Check sheet for the modelled part. Datum: model origin and axes. Units: mm. Give positions to 0.01 mm unless a question says otherwise; leave off trailing zeros. Loops run counter-clockwise (first coordinate to the right, second up) from the corner with the lowest first, then second, coordinate; pieces in that order, holes last. Notation, with made-up numbers: (-28, -37.5) -> (7, -37.5) arc R21 cw to (7, -29.5) -> close; hole circle Ø10 at (44, 23). An arc over 180 degrees is marked (long way). Write each question's results on one line, items separated by ' | '. Start each with the question number.
1. Cross-section at D-D on x = 78. Record the boundary of the cut face in (y, z).
2. Gauge pin test, flat ends, axial feed: pin 1 Ø1.5 at (y, z) = (6.5, -59) entering from +X; pin 2 Ø12 at (x, z) = (82, 32) entering from +Y; pin 3 Ø2.5 at (x, y) = (24, 4) entering from +Z; pin 4 Ø4 at (y, z) = (4.5, 27) entering from -X. Record the tip position at first contact, or that the pin passes through.
3. Material ranges on L1, parallel to X at y = 5, z = 17.5; L2, parallel to X at y = 1.75, z = -39; L3, parallel to Z at x = 23, y = 1.25, recorded low to high. Write a range as from..to.
4. Cross-section at C-C on x = -32.5. Record the boundary of the cut face in (y, z).
5. Cross-section at B-B on z = 0. Record the boundary of the cut face in (x, y).
6. Cross-section at A-A on x = 0. Record the boundary of the cut face in (y, z), and give its area (3 significant figures).
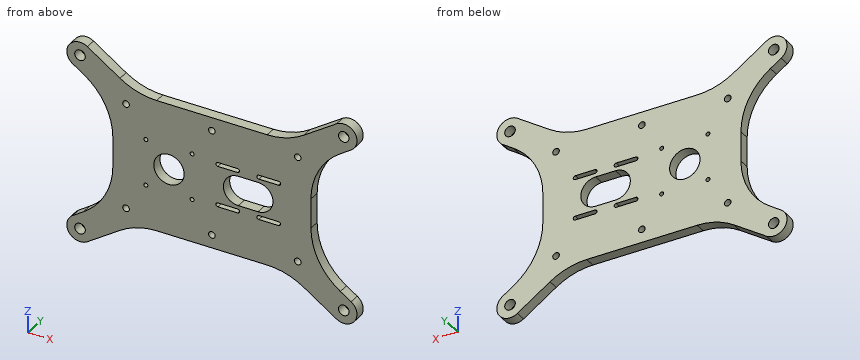
from build123d import *

# Parameters (mm, degrees)
SKETCH1_R           = 4
SKETCH1_R_2         = 11.5
BOSS_EXTRUDE1_DEPTH = 8
SKETCH2_R           = 2.5
SKETCH2_R_2         = 1.5
CUT_EXTRUDE1_DEPTH  = 8
FILLET1_R           = 50
FILLET2_R           = 50
CUT_EXTRUDE2_START  = -8
CUT_EXTRUDE2_DEPTH  = 8


# Read off the part's stored shape, not the designer's step: Cut-Extrude2
with BuildPart() as part:
    # Sketch1 → Boss-Extrude1 (new body)
    with BuildSketch(Plane(origin=(0, 0, 0), x_dir=(1, 0, 0), z_dir=(0, 1, 0))):
        with BuildLine():
            Line((105.393037283, -58.243520604), (75, -37.981495748))
            Line((75, -37.981495748), (75, 37.981495748))
            Line((75, 37.981495748), (105.393037283, 58.243520604))
            ThreePointArc((105.393037283, 58.243520604), (108.166538264, 72.111025509), (94.299033358, 74.88452649))
            Line((94.299033358, 74.88452649), (56.972243623, 50))
            Line((56.972243623, 50), (-56.972243623, 50))
            Line((-56.972243623, 50), (-94.299033358, 74.88452649))
            ThreePointArc((-94.299033358, 74.88452649), (-108.166538264, 72.111025509), (-105.393037283, 58.243520604))
            Line((-105.393037283, 58.243520604), (-75, 37.981495748))
            Line((-75, 37.981495748), (-75, -37.981495748))
            Line((-75, -37.981495748), (-105.393037283, -58.243520604))
            ThreePointArc((-105.393037283, -58.243520604), (-108.166538264, -72.111025509), (-94.299033358, -74.88452649))
            Line((-94.299033358, -74.88452649), (-56.972243623, -50))
            Line((-56.972243623, -50), (56.972243623, -50))
            Line((56.972243623, -50), (94.299033358, -74.88452649))
            ThreePointArc((94.299033358, -74.88452649), (108.166538264, -72.111025509), (105.393037283, -58.243520604))
        make_face()
        with Locations(Location((-99.846035321, -66.564023547, 0), (0, 0, 270))):
            Circle(SKETCH1_R, mode=Mode.SUBTRACT)
        with Locations(Location((-32.5, 0, 0), (0, 0, 270))):
            Circle(SKETCH1_R_2, mode=Mode.SUBTRACT)
        with Locations(Location((99.846035321, -66.564023547, 0), (0, 0, 270))):
            Circle(SKETCH1_R, mode=Mode.SUBTRACT)
        with Locations(Location((-99.846035321, 66.564023547, 0), (0, 0, 270))):
            Circle(SKETCH1_R, mode=Mode.SUBTRACT)
        with Locations(Location((99.846035321, 66.564023547, 0), (0, 0, 270))):
            Circle(SKETCH1_R, mode=Mode.SUBTRACT)
    extrude(amount=BOSS_EXTRUDE1_DEPTH)

    # Sketch2 → Cut-Extrude1 (cut)
    with BuildSketch(Plane(origin=(0, 8, 0), x_dir=(1, 0, 0), z_dir=(0, 1, 0))):
        with Locations(Location((-65, 40, 0), (0, 0, 270))):
            Circle(SKETCH2_R)
        with Locations(Location((65, 40, 0), (0, 0, 270))):
            Circle(SKETCH2_R)
        with Locations(Location((65, -40, 0), (0, 0, 270))):
            Circle(SKETCH2_R)
        with Locations(Location((-65, -40, 0), (0, 0, 270))):
            Circle(SKETCH2_R)
        with Locations(Location((0, -40, 0), (0, 0, 270))):
            Circle(SKETCH2_R)
        with Locations(Location((0, 40, 0), (0, 0, 270))):
            Circle(SKETCH2_R)
        with Locations(Location((-15, 17.5, 0), (0, 0, 270))):
            Circle(SKETCH2_R_2)
        with Locations(Location((-50, 17.5, 0), (0, 0, 270))):
            Circle(SKETCH2_R_2)
        with Locations(Location((-50, -17.5, 0), (0, 0, 270))):
            Circle(SKETCH2_R_2)
        with Locations(Location((-15, -17.5, 0), (0, 0, 270))):
            Circle(SKETCH2_R_2)
    extrude(amount=-CUT_EXTRUDE1_DEPTH, mode=Mode.SUBTRACT)

    # Fillet1
    fillet1_edges = [part.edges().sort_by_distance(p)[0] for p in [
        (-56.972243623, 4, -50),
        (56.972243623, 4, -50),
        (56.972243623, 4, 50),
        (-56.972243623, 4, 50),
    ]]
    fillet(fillet1_edges, radius=FILLET1_R)

    # Fillet2
    fillet2_edges = [part.edges().sort_by_distance(p)[0] for p in [
        (75, 4, -37.981495748),
        (75, 4, 37.981495748),
        (-75, 4, 37.981495748),
        (-75, 4, -37.981495748),
    ]]
    fillet(fillet2_edges, radius=FILLET2_R)

    # Cut-Extrude2 outline → Cut-Extrude2 (cut)
    with BuildSketch(Plane(origin=(0, 8, 0), x_dir=(1, 0, 0), z_dir=(0, 1, 0)).offset(CUT_EXTRUDE2_START)):
        with BuildLine():
            Line((35, 11.25), (20, 11.25))
            ThreePointArc((20, 11.25), (8.75, 0), (20, -11.25))
            Line((20, -11.25), (35, -11.25))
            ThreePointArc((35, -11.25), (46.25, 0), (35, 11.25))
        make_face()
        with BuildLine():
            ThreePointArc((35.5, 17), (34, 15.5), (35.5, 14))
            Line((35.5, 14), (50.5, 14))
            ThreePointArc((50.5, 14), (52, 15.5), (50.5, 17))
            Line((50.5, 17), (35.5, 17))
        make_face()
        with BuildLine():
            ThreePointArc((4.5, 17), (3, 15.5), (4.5, 14))
            Line((4.5, 14), (19.5, 14))
            ThreePointArc((19.5, 14), (21, 15.5), (19.5, 17))
            Line((19.5, 17), (4.5, 17))
        make_face()
        with BuildLine():
            ThreePointArc((4.5, -14), (3, -15.5), (4.5, -17))
            Line((4.5, -17), (19.5, -17))
            ThreePointArc((19.5, -17), (21, -15.5), (19.5, -14))
            Line((19.5, -14), (4.5, -14))
        make_face()
        with BuildLine():
            ThreePointArc((35.5, -14), (34, -15.5), (35.5, -17))
            Line((35.5, -17), (50.5, -17))
            ThreePointArc((50.5, -17), (52, -15.5), (50.5, -14))
            Line((50.5, -14), (35.5, -14))
        make_face()
    extrude(amount=CUT_EXTRUDE2_DEPTH, mode=Mode.SUBTRACT)


solid = part.part
Geometry says:
1) outline: (0, -64.02) -> (8, -64.02) -> (8, -28.28) -> (0, -28.28) -> close; (0, 28.28) -> (8, 28.28) -> (8, 64.02) -> (0, 64.02) -> close
2) pin 1: x = 107.17 | pin 2: y = 8 | pin 3: z = 50 | pin 4: x = -78.27
3) L1: -75.4..-51.5, -48.5..-16.5, -13.5..75.4 | L2: -83.43..-67.29, -62.71..-2.29, 2.29..62.71, 67.29..83.43 | L3: -50..-11.25, 11.25..50
4) outline: (0, -50) -> (8, -50) -> (8, -11.5) -> (0, -11.5) -> close; (0, 11.5) -> (8, 11.5) -> (8, 50) -> (0, 50) -> close
5) outline: (-75, 0) -> (-44, 0) -> (-44, 8) -> (-75, 8) -> close; (-21, 0) -> (8.75, 0) -> (8.75, 8) -> (-21, 8) -> close; (46.25, 0) -> (75, 0) -> (75, 8) -> (46.25, 8) -> close
6) outline: (0, -50) -> (8, -50) -> (8, -42.5) -> (0, -42.5) -> close; (0, -37.5) -> (8, -37.5) -> (8, 37.5) -> (0, 37.5) -> close; (0, 42.5) -> (8, 42.5) -> (8, 50) -> (0, 50) -> close | area: 720 mm^2
